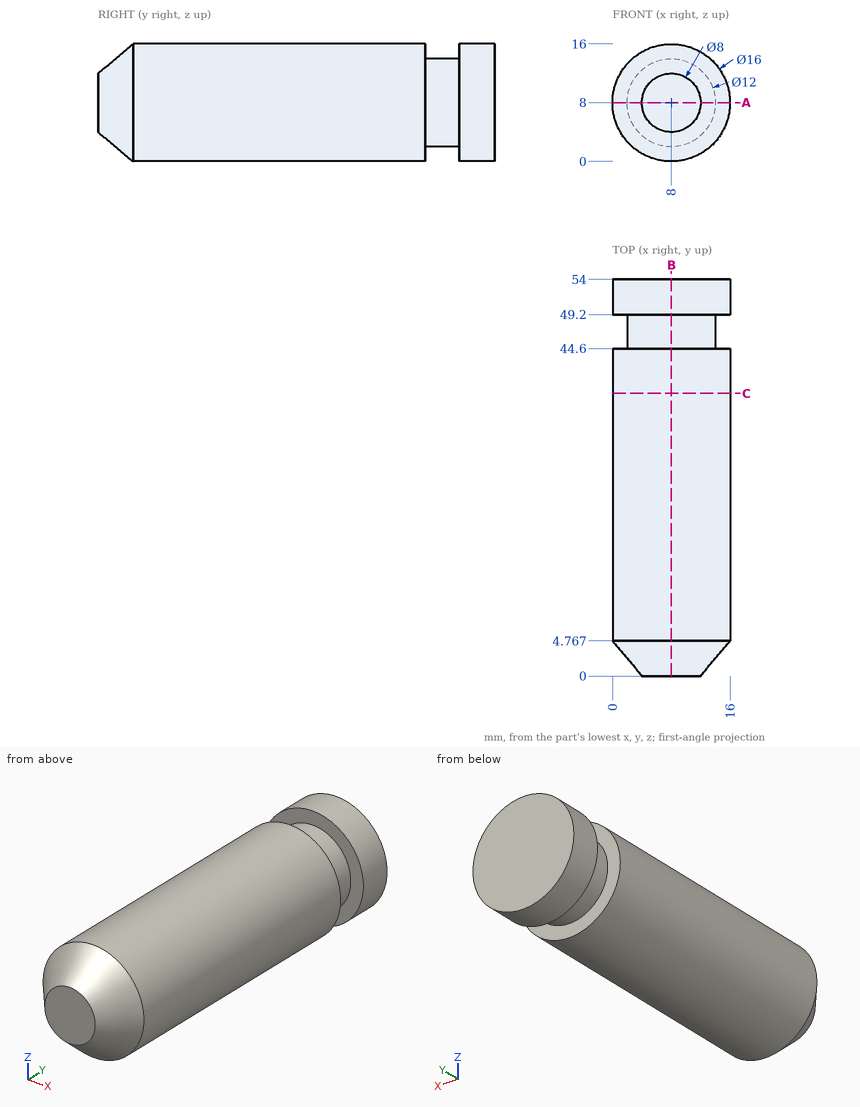
Could you check a few things on this drawing? It's one solid part, dimensions in mm from its lowest x, y, z. Coordinates: 2 decimals unless noted, no trailing zeros. Order: outer loops, then holes, each group sorted by start corner. A loop starts at its lowest first (then second) coordinate and runs counter-clockwise, first axis right, second up.
1) Imagine slicing it at A-A on z = 8. List the corners of the cut face in (x, y) for me, and give its area (3 significant figures).
2) Will these pins go through, and if not, where does the flat tip stop? pin 1 (4 mm diameter, centred on y = 14, z = 11.5, fed in from -X); pin 2 (4 mm diameter, centred on y = 48.5, z = 2, fed in from -X).
3) Imagine slicing it at C-C on y = 38.5. List the corners of the cut face in (x, z) for me, and give its area (3 significant figures).
4) I need wall thicknesses on line 1 (Z direction, x = 1.5, y = 30); line 2 (Y direction, x = 5.5, z = 13.25); line 3 (Z direction, x = 10.25, y = 38.5). Which ranges of each line are inside material? Lowest first, please.
5) Imagine slicing it at B-B on x = 8. List the corners of the cut face in (y, z) for me, and give its area (3 significant figures).
Response values:
1. outline: (0, 4.77) - (4, 0) - (12, 0) - (16, 4.77) - (16, 44.6) - (14, 44.6) - (14, 49.2) - (16, 49.2) - (16, 54) - (0, 54) - (0, 49.2) - (2, 49.2) - (2, 44.6) - (0, 44.6) - close
1. area: 827 mm2
2. pin 1: stops at x = 0.14
2. pin 2: stops at x = 1.15
3. outline: circle Ø16 at (8, 8)
3. area: 201 mm2
4. line 1: z = 3.34 to 12.66
4. line 2: y = 2.16 to 54
4. line 3: z = 0.32 to 15.68
5. outline: (0, 4) - (4.77, 0) - (44.6, 0) - (44.6, 2) - (49.2, 2) - (49.2, 0) - (54, 0) - (54, 16) - (49.2, 16) - (49.2, 14) - (44.6, 14) - (44.6, 16) - (4.77, 16) - (0, 12) - close
5. area: 827 mm2
